Here's how the part is built. I have some questions about the finished solid (model axes, mm). A direction names the side the tool comes from. Give positions to 0.01 mm unless a question says otherwise; leave off trailing zeros. Write each loop counter-clockwise with the first axis right and the second up, starting at its lowest first coordinate (ties: lowest second). Pieces come first, ordered by that corner, then holes. Notation, with made-up numbers: (55, -9) - (90, -9) arc R17 ccw to (90, 14) - close; hole circle Ø7 at (83, 19). An arc over 180 degrees is marked (long way). One line per item, written item: value. Start each with the question number.
1) Imagine slicing it at A-A on x = -170. Write out the boundary of the cut face in (y, z), plus the area to 3 significant figures.
2) Imagine slicing it at C-C on z = -92.5. Write out the boundary of the cut face in (x, y).
3) I'm going to push flat-ended pins straight in: P1, Ø1.5, axis at y = 7, z = -52.5, coming from the +X side; P2, Ø9.5, axis at x = -202.25, z = -146.95, coming from the -Y side. Where does each tip first touch, or does it pass through?
4) We'd pull the mould along Z, two halves only. Please class faces 3 (the flat face through (0, 6, -277)), 4 (the flat face through (-148, 6, 300)), 5 (the cylindrical face through (-48.074, 5.916, -194.136)): +Z half, -Z half, draft (parallel to the pull), parting line (faces both ways), or undercut.
5) On a 3-axis mill with a long thin cutter (end or side, diameter ignored), from which of +Z, -Z, +X, -X, +Y, -Y can I reach the whole of each face in a straight line? I mean faces 1 (the flat face through (0, 6, 238)), 2 (the flat face through (-140.317, 5.916, -151.687)). Say none if no direction works.
6) Imagine slicing it at D-D on z = 127. Write out the boundary of the cut face in (x, y), plus the area to 3 significant figures.
7) Imagine slicing it at B-B on y = 6. Count the separate pieces of the cut face and the enclosed holes in it, plus the area to 3 significant figures.
8) Please list where these lines run through material, in increasing order: L1, parallel to Z at x = -250, y = 6; L2, parallel to X at y = 4.75, z = 0; L3, parallel to X at y = 10, z = 94.5. Write a range as [from, to].
from build123d import *

# Parameters (mm, degrees)
SKETCH1_R           = 3
SKETCH1_R_2         = 1.5
BOSS_EXTRUDE1_DEPTH = 12


with BuildPart() as part:
    # Sketch1 → Boss-Extrude1 (new body)
    with BuildSketch(Plane(origin=(0, 0, 0), x_dir=(1, 0, 0), z_dir=(0, 1, 0))):
        with BuildLine():
            Line((-203.190468868, 99.063784307), (-199.902587408, -6.241437954))
            ThreePointArc((-199.902587408, -6.241437954), (-173.205080757, -100), (-105.356537529, -170))
            Line((-105.356537529, -170), (-15.803480629, -225.5))
            ThreePointArc((-15.803480629, -225.5), (-8.215838363, -228.853076093), (0, -230))
            Line((0, -230), (0, -247))
            ThreePointArc((0, -247), (-3, -250), (0, -253))
            Line((0, -253), (0, -300))
            Line((0, -300), (-300, -300))
            Line((-300, -300), (-300, 300))
            Line((-300, 300), (0, 300))
            Line((0, 300), (0, 253))
            ThreePointArc((0, 253), (-3, 250), (0, 247))
            Line((0, 247), (0, 200))
            ThreePointArc((0, 200), (-48.742755406, 193.969440365), (-94.546049879, 176.241437954))
            Line((-94.546049879, 176.241437954), (-187.386988239, 126.436215693))
            ThreePointArc((-187.386988239, 126.436215693), (-199.18584287, 115), (-203.190468868, 99.063784307))
        make_face()
        with Locations(Location((-77.254248594, -237.764129074, 0), (0, 0, 270))):
            Circle(SKETCH1_R, mode=Mode.SUBTRACT)
        with Locations(Location((-146.946313073, -202.254248594, 0), (0, 0, 270))):
            Circle(SKETCH1_R, mode=Mode.SUBTRACT)
        with Locations(Location((-202.254248594, -146.946313073, 0), (0, 0, 270))):
            Circle(SKETCH1_R, mode=Mode.SUBTRACT)
        with Locations(Location((-237.764129074, -77.254248594, 0), (0, 0, 270))):
            Circle(SKETCH1_R, mode=Mode.SUBTRACT)
        with Locations(Location((-250, 0, 0), (0, 0, 270))):
            Circle(SKETCH1_R, mode=Mode.SUBTRACT)
        with Locations(Location((-237.764129074, 77.254248594, 0), (0, 0, 270))):
            Circle(SKETCH1_R, mode=Mode.SUBTRACT)
        with Locations(Location((-202.254248594, 146.946313073, 0), (0, 0, 270))):
            Circle(SKETCH1_R, mode=Mode.SUBTRACT)
        with Locations(Location((-146.946313073, 202.254248594, 0), (0, 0, 270))):
            Circle(SKETCH1_R, mode=Mode.SUBTRACT)
        with Locations(Location((-77.254248594, 237.764129074, 0), (0, 0, 270))):
            Circle(SKETCH1_R, mode=Mode.SUBTRACT)
        with Locations(Location((-250, 250, 0), (0, 0, 270))):
            Circle(SKETCH1_R_2, mode=Mode.SUBTRACT)
        with Locations(Location((-250, -250, 0), (0, 0, 270))):
            Circle(SKETCH1_R_2, mode=Mode.SUBTRACT)
    extrude(amount=BOSS_EXTRUDE1_DEPTH)


solid = part.part
Numbers:
1. outline: (0, -300) - (12, -300) - (12, -135.76) - (0, -135.76) - close; (0, 105.36) - (12, 105.36) - (12, 300) - (0, 300) - close
1. area: 4,310 mm^2
2. outline: (-300, 0) - (-202.99, 0) - (-202.99, 12) - (-300, 12) - close
3. P1: x = -201.71
3. P2: y = 0
4. face 3: draft
4. face 4: +Z half
4. face 5: undercut
5. face 1: +Z, -Z, +X, +Y, -Y
5. face 2: +X, +Y, -Y
6. outline: (-300, 0) - (-154.5, 0) - (-154.5, 12) - (-300, 12) - close
6. area: 1,750 mm^2
7. separate pieces: 1
7. enclosed holes: 11
7. area: 113,000 mm^2
8. L1: [-300, -251.5], [-248.5, -3], [3, 248.5], [251.5, 300]
8. L2: [-300, -253], [-247, -200.1]
8. L3: [-300, -176.27]
